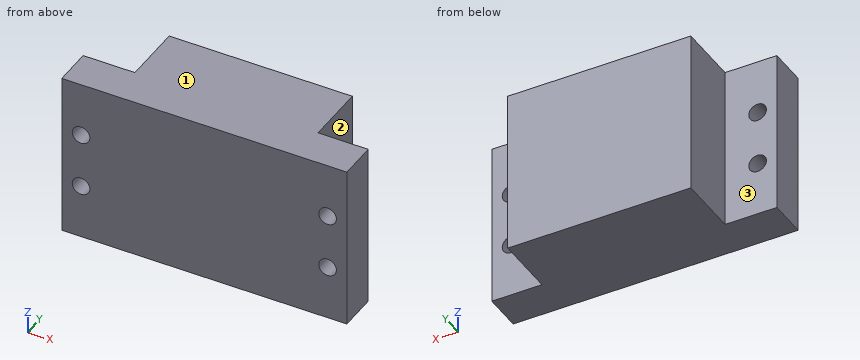
from build123d import *

# Parameters (mm, degrees)
SKETCH1_W           = 80.772
SKETCH1_H           = 46.7
BOSS_EXTRUDE1_DEPTH = 10.9
SKETCH3_R           = 2.5
CUT_EXTRUDE1_DEPTH  = 10.9
SKETCH8_W           = 51.8805497
SKETCH8_H           = 46.7
BOSS_EXTRUDE2_DEPTH = 17.5


with BuildPart() as part:
    # Sketch1 → Boss-Extrude1 (new body)
    with BuildSketch(Plane(origin=(0, 0, 0), x_dir=(1, 0, 0), z_dir=(0, 1, 0))):
        with Locations((4.445313725, -13.27745098)):
            Rectangle(SKETCH1_W, SKETCH1_H)
    extrude(amount=BOSS_EXTRUDE1_DEPTH)

    # Sketch3 → Cut-Extrude1 (cut)
    with BuildSketch(Plane(origin=(0, 10.9, 0), x_dir=(1, 0, 0), z_dir=(0, 1, 0))):
        with Locations(Location((-30.479686275, -5.42745098, 0), (0, 0, 270))):
            Circle(SKETCH3_R)
        with Locations(Location((-30.479686275, -21.12745098, 0), (0, 0, 270))):
            Circle(SKETCH3_R)
        with Locations(Location((39.370313725, -5.42745098, 0), (0, 0, 270))):
            Circle(SKETCH3_R)
        with Locations(Location((39.370313725, -21.12745098, 0), (0, 0, 270))):
            Circle(SKETCH3_R)
    extrude(amount=-CUT_EXTRUDE1_DEPTH, mode=Mode.SUBTRACT)

    # Sketch8 → Boss-Extrude2 (add)
    with BuildSketch(Plane(origin=(0, 10.9, 0), x_dir=(1, 0, 0), z_dir=(0, 1, 0))):
        with Locations((4.667038875, -13.27745098)):
            Rectangle(SKETCH8_W, SKETCH8_H)
    extrude(amount=BOSS_EXTRUDE2_DEPTH)


solid = part.part
Could you check a few things on this model? Use its own coordinates, in mm. Face numbers are marked on the shaded views. A direction names the side the tool comes from. Coordinates: 2 decimals unless noted, no trailing zeros. Write each loop counter-clockwise with the first axis right and the second up, starting at its lowest first coordinate (ties: lowest second). Pieces come first, ordered by that corner, then holes. Notation, with made-up numbers: (57, -6) - (71, -6) arc R30 cw to (71, 32) - close; hole circle Ø3 at (45.5, 66). An arc over 180 degrees is marked (long way). Write item = value, one per line.
1) Suppose I cut it at A-A on x = 40.5. Please give me the cut outline in (y, z), plus the area to 3 significant figures.
Result set:
outline = (0, -10.07) - (10.9, -10.07) - (10.9, 3.2) - (0, 3.2) - close; (0, 7.66) - (10.9, 7.66) - (10.9, 18.9) - (0, 18.9) - close; (0, 23.36) - (10.9, 23.36) - (10.9, 36.63) - (0, 36.63) - close
area = 412 mm2
2) For the marked faces 1, 2 and 3, which set-ups out of +Z, -Z, +X, -X, +Y, -Y let a thin tool reach every point of the face, with its end or its side?
Result set:
face_1 = +Z, +X, -X, +Y, -Y
face_2 = +Z, -Z, +X, +Y
face_3 = +Z, -Z, -X, +Y
3) Suppose I cut it at B-B on z = 12. Please give me the cut outline in (x, y), plus the area to 3 significant figures.
Result set:
outline = (-35.94, 0) - (44.83, 0) - (44.83, 10.9) - (30.61, 10.9) - (30.61, 28.4) - (-21.27, 28.4) - (-21.27, 10.9) - (-35.94, 10.9) - close
area = 1,790 mm2
4) Suppose I cut it at C-C on y = 2.25. Please give me the cut outline in (x, z), plus the area to 3 significant figures.
Result set:
outline = (-35.94, -10.07) - (44.83, -10.07) - (44.83, 36.63) - (-35.94, 36.63) - close; hole circle Ø5 at (-30.48, 5.43); hole circle Ø5 at (-30.48, 21.13); hole circle Ø5 at (39.37, 5.43); hole circle Ø5 at (39.37, 21.13)
area = 3,690 mm2
5) Suppose I cut it at D-D on z = 21. Please give me the cut outline in (x, y), plus the area to 3 significant figures.
Result set:
outline = (-35.94, 0) - (-32.98, 0) - (-32.98, 10.9) - (-35.94, 10.9) - close; (-27.98, 0) - (36.87, 0) - (36.87, 10.9) - (30.61, 10.9) - (30.61, 28.4) - (-21.27, 28.4) - (-21.27, 10.9) - (-27.98, 10.9) - close; (41.87, 0) - (44.83, 0) - (44.83, 10.9) - (41.87, 10.9) - close
area = 1,680 mm2
6) Please list where these lines run through material, in increasing order: line 1 (X direction, y = 8.75, z = 5.5); line 2 (Y direction, x = 35, z = 12); line 3 (X direction, y = 23.75, z = 18). Write a range as [from, to].
Result set:
line_1 = [-35.94, -32.98], [-27.98, 36.87], [41.87, 44.83]
line_2 = [0, 10.9]
line_3 = [-21.27, 30.61]
7) Will these pins go through, and if not, where does the flat tip stop? pin 1 Ø3 at (x, z) = (-27.5, -0.5) entering from +Y; pin 2 Ø10 at (y, z) = (19.5, 25.5) entering from +X; pin 3 Ø9 at (y, z) = (23.5, 19) entering from -X.
Result set:
pin_1 = 10.9
pin_2 = 30.61
pin_3 = -21.27
